Solid Edge part; units mm, degrees
sketch "Sketch1" plane through (0, 0, 0) normal (1, 0, 0) x (0, 1, 0)
  arc A0 (0, 48) -> (-48, 0) centre (0, 0) ccw
  line L0 (-48, 0) -> (0, 0)
  line L1 (0, 0) -> (0, 48)
extrude "Protrusion1" add sketch "Sketch1" along normal blind 16
sketch "Sketch2" plane through (0, 0, 0) normal (1, 0, 0) x (0, 1, 0)
  line L0 (-48, -16) -> (-48, 0)
  line L1 (-48, 0) -> (0, 0)
  line L2 (0, 0) -> (0, -16)
  line L3 (0, -16) -> (-48, -16)
extrude "ExtrudedProtrusion_2" add sketch "Sketch2" along normal blind 96
sketch "Sketch3" plane through (0, 0, 0) normal (1, 0, 0) x (0, 1, 0)
  line L0 (0, 48) -> (0, 28)
  line L1 (0, 28) -> (16, 28)
  line L2 (16, 28) -> (16, 48)
  line L3 (16, 48) -> (0, 48)
extrude "Protrusion_3" add sketch "Sketch3" along normal blind 16
sketch "Sketch4" plane through (0, 0, 0) normal (1, 0, 0) x (0, 1, 0)
  line L0 (0, -16) -> (0, 28)
  line L1 (0, 28) -> (16, 28)
  line L2 (16, 28) -> (16, -16)
  line L3 (16, -16) -> (0, -16)
extrude "Protrusion_4" add sketch "Sketch4" along normal blind 96
sketch "Sketch5" plane through (56, 0, 14) normal (0, -1, 0) x (1, 0, 0)
  line L0 (0, -14) -> (0, 14)
  line L1 (0, 14) -> (40, 14)
  line L2 (40, 14) -> (40, -14)
  line L3 (40, -14) -> (0, -14)
extrude "Cutout_1" cut sketch "Sketch5" against normal blind 4
sketch "Sketch6" plane through (76, 4, 14) normal (0, -1, 0) x (1, 0, 0)
  line L0 (20, -14) -> (-20, 14)
  line L1 (-20, 14) -> (20, 14)
  line L2 (20, 14) -> (20, -14)
extrude "Cutout_2" cut sketch "Sketch6" against normal blind 12
sketch "Sketch7" plane through (36, 0, 14) normal (0, -1, 0) x (1, 0, 0)
  line L0 (-20, -14) -> (-20, 14)
  line L1 (20, -14) -> (-20, -14)
  line L2 (20, 14) -> (20, -14)
  line L3 (-20, 14) -> (20, 14)
extrude "Protrusion_5" add sketch "Sketch7" along normal blind 10
sketch "Sketch8" plane through (36, -10, 14) normal (0, -1, 0) x (1, 0, 0)
  line L0 (12, 14) -> (-12, 14)
  arc A0 (-12, 14) -> (12, 14) centre (0, 14) ccw
extrude "Cutout_3" cut sketch "Sketch8" against normal blind 26
sketch "Sketch9" plane through (56, -22, 0) normal (0, 0, 1) x (1, 0, 0)
  line L0 (40, 6) -> (20, 6)
  arc A0 (20, 6) -> (20, -10) centre (20, -2) ccw
  line L1 (40, -10) -> (20, -10)
  line L2 (40, 6) -> (40, -10)
extrude "Cutout_4" cut sketch "Sketch9" against normal blind 16
sketch "Sketch10" plane through (36, -10, 14) normal (0, -1, 0) x (1, 0, 0)
  line L0 (-20, -14) -> (-20, 13.9689)
  line L1 (-20, 13.9689) -> (-12, 14)
  arc A0 (-12, 14) -> (12, 14) centre (0, 14.0466) ccw
  line L2 (20, 14) -> (12, 14)
  line L3 (20, 14) -> (20, -14)
  line L4 (20, -14) -> (-20, -14)
extrude "Protrusion_6" add sketch "Sketch10" against normal blind 26
sketch "Sketch11" plane through (36, -10, 14) normal (0, -1, 0) x (1, 0, 0)
  line L0 (20, 14) -> (12, 14)
  line L1 (20, -14) -> (20, 14)
  line L2 (-20, -14) -> (20, -14)
  line L3 (-20, 14) -> (-20, -14)
  line L4 (-12, 14) -> (-20, 14)
  arc A0 (-12, 14) -> (12, 14) centre (0, 14) ccw
extrude "Protrusion2" add sketch "Sketch11" along normal blind 16
Work out the finished part from the listing and answer in its coordinate system (mm). A direction names the side the tool comes from. Give positions to 0.01 mm unless a question says otherwise; leave off trailing zeros. Loops run counter-clockwise (first coordinate to the right, second up) from the corner with the lowest first, then second, coordinate; pieces in that order, holes last. Notation, with made-up numbers: M 31.5,17.25 L 36.5,17.25 A13 ccw 36.5,25.25 Z; hole C 32.25,28.25 d1. An arc over 180 degrees is marked long. Use CSV: the item, a comma, the result in double quotes.
1) Find section A-A on x = 85.5. Write down the section's boundary in (y, z), plus the area to 3 significant figures.
Answer:
outline,"M -48,-16 L -32,-16 L -32,0 L -48,0 Z; M -16,-16 L 16,-16 L 16,7.35 L 4,7.35 L 4,0 L -16,0 Z"
area,"856 mm^2"
2) Given P1, Ø4, axis at x = 20, y = -10, coming from the +Z side, flat-ended and moving along its own axis, determine where the tip first touches the part or whether it passes through.
Answer:
P1,"z = 28"
3) Find section D-D on z = -10.5. Write down the section's boundary in (x, y), plus the area to 3 significant figures.
Answer:
outline,"M 0,-48 L 96,-48 L 96,-32 L 76,-32 A8 cw 76,-16 L 96,-16 L 96,16 L 0,16 Z"
area,"5,720 mm^2"
4) Determine the mould class of faces 6 (the flat face through (76, 10, 14)), 7 (the cylindrical face through (36, -18, 16)), 8 (the cylindrical face through (35.74, 2.82, 16.05)), 9 (the flat face through (55, -28, 0)) for opening direction X: released by +X, released by -X, zero draft, split by the parting line, or undercut.
Answer:
face 6,"released by +X"
face 7,"undercut"
face 8,"undercut"
face 9,"zero draft"
5) Consider L1, parallel to Y at x = 85, z = -4.5; L2, parallel to Z at x = 35.5, y = -29; L3, parallel to X at y = -30.5, z = 29. Determine where each line is inside the solid, lowest interval first.
Answer:
L1,"-48 to -32, -16 to 16"
L2,"-16 to 0"
L3,"0 to 16"
6) Find section C-C on x = 36. Write down the section's boundary in (y, z).
Answer:
outline,"M -48,-16 L 16,-16 L 16,16.05 L -10,16.05 L -10,16 L -26,16 L -26,0 L -48,0 Z"
7) Which of the six approach directions +Z, -Z, +X, -X, +Y, -Y give full straight-line access (tool end or side, diameter ignored) to faces 1 (the flat face through (8, 8, 48)), 2 (the flat face through (56, -11, 14)), 3 (the flat face through (86, -16, -8)), 4 (the flat face through (52, -18, 28)), 5 (the flat face through (37, 16, 8))?
Answer:
face 1,"+Z, +X, -X, +Y, -Y"
face 2,"+Z, +X, -Y"
face 3,"+Z, -Z, +X"
face 4,"+Z, +X, +Y, -Y"
face 5,"+Z, -Z, +X, -X, +Y"
